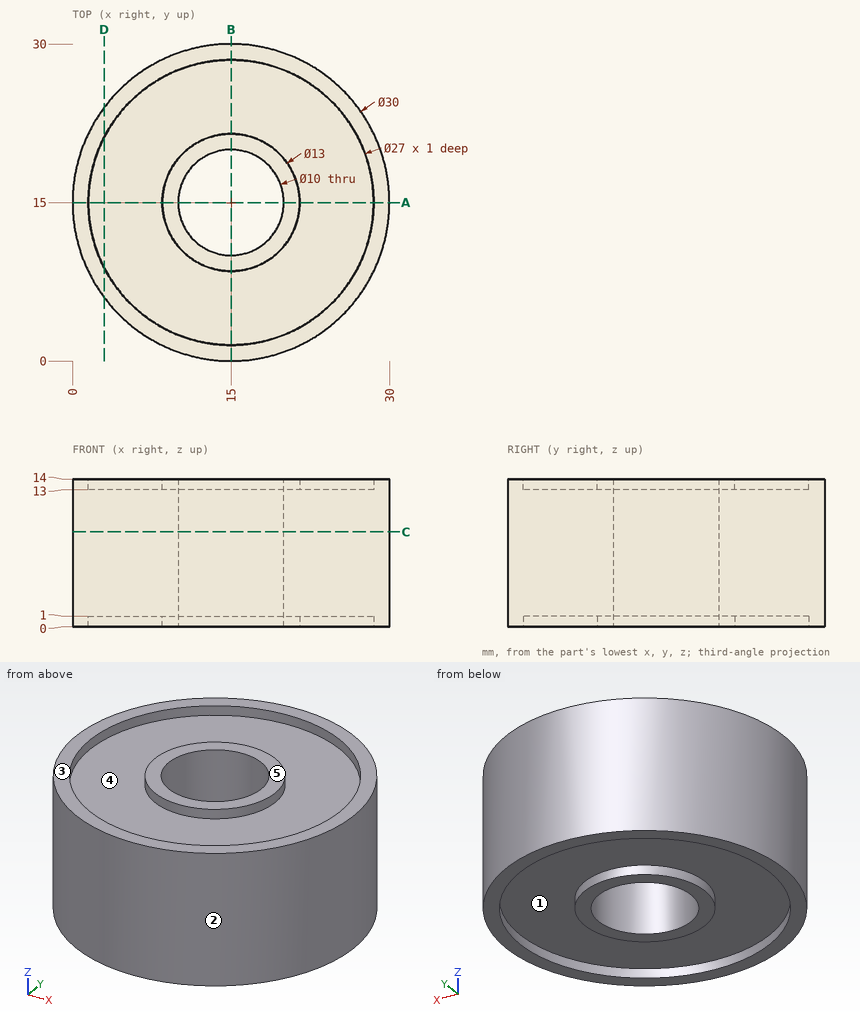
Study the drawing (mm; zero at the part's minimum x, y, z) and answer. A direction names the side the tool comes from. Give positions to 0.01 mm unless a question says otherwise; leave off trailing zeros. Loops run counter-clockwise (first coordinate to the right, second up) from the corner with the lowest first, then second, coordinate; pieces in that order, holes last. Notation, with made-up numbers: (17, 67) -> (43, 67) arc R20 ccw to (43, 91) -> close; hole circle Ø6 at (42.5, 42.25). An arc over 180 degrees is marked (long way). Write item = value, one per line. Start each with the question number.
(1) Find the intervals of material crossed by probe 1 along Y at (x, z) = (15, 0.8); probe 2 along Y at (x, z) = (15, 6.5); probe 3 along Z at (x, y) = (24.75, 12), in increasing order. Write a range as from..to.
(2) Given pin 1 Ø10 at (x, y) = (4.5, 8.5) entering from -Z; pin 2 Ø6 at (x, z) = (24, 10.5) entering from -Y; pin 3 Ø1 at (y, z) = (9, 11) entering from -X; pin 4 Ø2 at (x, z) = (23.5, 7.5) entering from -Y, each flat-ended and moving along its own axis, determine where each tip first touches the part or whether it passes through.
(3) Find section A-A on y = 15. Give the vertices of the cut face in (x, z), and give its area (3 significant figures).
(4) Find section D-D on x = 3. Give the vertices of the cut face in (y, z), and give its area (3 significant figures).
(5) The mould has two halves that part along X. Classify the marked faces 1, 2 and 3: +X half, -X half, draft (parallel to the pull), parting line (faces both ways), or undercut.
(6) Which of the six approach directions +Z, -Z, +X, -X, +Y, -Y give full straight-line access (tool end or side, diameter ignored) to the marked faces 4 and 5?
(7) Find section C-C on z = 9. Give the vertices of the cut face in (x, y), and give its area (3 significant figures).
From the geometry:
q1.probe_1 = 0..1.5, 8.5..10, 20..21.5, 28.5..30
q1.probe_2 = 0..10, 20..30
q1.probe_3 = 1..13
q2.pin_1 = 0
q2.pin_2 = 1.25
q2.pin_3 = 1.04
q2.pin_4 = 2.01
q3.outline = (0, 0) -> (1.5, 0) -> (1.5, 1) -> (8.5, 1) -> (8.5, 0) -> (10, 0) -> (10, 14) -> (8.5, 14) -> (8.5, 13) -> (1.5, 13) -> (1.5, 14) -> (0, 14) -> close; (20, 0) -> (21.5, 0) -> (21.5, 1) -> (28.5, 1) -> (28.5, 0) -> (30, 0) -> (30, 14) -> (28.5, 14) -> (28.5, 13) -> (21.5, 13) -> (21.5, 14) -> (20, 14) -> close
q3.area = 252 mm^2
q4.outline = (6, 0) -> (8.82, 0) -> (8.82, 1) -> (21.18, 1) -> (21.18, 0) -> (24, 0) -> (24, 14) -> (21.18, 14) -> (21.18, 13) -> (8.82, 13) -> (8.82, 14) -> (6, 14) -> close
q4.area = 227 mm^2
q5.face_1 = undercut
q5.face_2 = parting line
q5.face_3 = draft
q6.face_4 = +Z
q6.face_5 = +Z, +X, -X, +Y, -Y
q7.outline = circle Ø30 at (15, 15); hole circle Ø10 at (15, 15)
q7.area = 628 mm^2
